from build123d import *

# Parameters (mm, degrees)
SKETCH1_R           = 3.4
BOSS_EXTRUDE1_DEPTH = 400


with BuildPart() as part:
    # Sketch1 → Boss-Extrude1 (new body)
    with BuildSketch(Plane.XY):
        with BuildLine():
            Line((20, 17.75), (20, 5.15))
            Line((20, 5.15), (19, 5.15))
            Line((19, 5.15), (19, 4.15))
            Line((19, 4.15), (15.4, 4.15))
            Line((15.4, 4.15), (15.4, 6.35))
            Line((15.4, 6.35), (16.95, 6.35))
            ThreePointArc((16.95, 6.35), (17.833883476, 6.716116524), (18.2, 7.6))
            Line((18.2, 7.6), (18.2, 9.3))
            ThreePointArc((18.2, 9.3), (17.907106781, 10.007106781), (17.2, 10.3))
            Line((17.2, 10.3), (12.03669957, 10.3))
            ThreePointArc((12.03669957, 10.3), (11.73040037, 10.239040459), (11.470780817, 10.065452001))
            Line((11.470780817, 10.065452001), (6.084081247, 4.674305984))
            ThreePointArc((6.084081247, 4.674305984), (5.910833239, 4.414848262), (5.85, 4.108853983))
            Line((5.85, 4.108853983), (5.85, -4.108853983))
            ThreePointArc((5.85, -4.108853983), (5.910833239, -4.414848262), (6.084081247, -4.674305984))
            Line((6.084081247, -4.674305984), (11.470780817, -10.065452001))
            ThreePointArc((11.470780817, -10.065452001), (11.73040037, -10.239040459), (12.03669957, -10.3))
            Line((12.03669957, -10.3), (17.2, -10.3))
            ThreePointArc((17.2, -10.3), (17.907106781, -10.007106781), (18.2, -9.3))
            Line((18.2, -9.3), (18.2, -7.6))
            ThreePointArc((18.2, -7.6), (17.833883476, -6.716116524), (16.95, -6.35))
            Line((16.95, -6.35), (15.4, -6.35))
            Line((15.4, -6.35), (15.4, -4.15))
            Line((15.4, -4.15), (19, -4.15))
            Line((19, -4.15), (19, -5.15))
            Line((19, -5.15), (20, -5.15))
            Line((20, -5.15), (20, -17.75))
            ThreePointArc((20, -17.75), (19.340990258, -19.340990258), (17.75, -20))
            Line((17.75, -20), (5.15, -20))
            Line((5.15, -20), (5.15, -19))
            Line((5.15, -19), (4.15, -19))
            Line((4.15, -19), (4.15, -15.4))
            Line((4.15, -15.4), (6.35, -15.4))
            Line((6.35, -15.4), (6.35, -16.95))
            ThreePointArc((6.35, -16.95), (6.716116524, -17.833883476), (7.6, -18.2))
            Line((7.6, -18.2), (9.3, -18.2))
            ThreePointArc((9.3, -18.2), (10.007106781, -17.907106781), (10.3, -17.2))
            Line((10.3, -17.2), (10.3, -12.054477022))
            ThreePointArc((10.3, -12.054477022), (10.239166761, -11.748482743), (10.065918753, -11.489025021))
            Line((10.065918753, -11.489025021), (4.665899173, -6.084547999))
            ThreePointArc((4.665899173, -6.084547999), (4.406279619, -5.910959541), (4.09998042, -5.85))
            Line((4.09998042, -5.85), (-4.09998042, -5.85))
            ThreePointArc((-4.09998042, -5.85), (-4.406279619, -5.910959541), (-4.665899173, -6.084547999))
            Line((-4.665899173, -6.084547999), (-10.065918753, -11.489025021))
            ThreePointArc((-10.065918753, -11.489025021), (-10.239166761, -11.748482743), (-10.3, -12.054477022))
            Line((-10.3, -12.054477022), (-10.3, -17.2))
            ThreePointArc((-10.3, -17.2), (-10.007106781, -17.907106781), (-9.3, -18.2))
            Line((-9.3, -18.2), (-7.6, -18.2))
            ThreePointArc((-7.6, -18.2), (-6.716116524, -17.833883476), (-6.35, -16.95))
            Line((-6.35, -16.95), (-6.35, -15.4))
            Line((-6.35, -15.4), (-4.15, -15.4))
            Line((-4.15, -15.4), (-4.15, -19))
            Line((-4.15, -19), (-5.15, -19))
            Line((-5.15, -19), (-5.15, -20))
            Line((-5.15, -20), (-17.75, -20))
            ThreePointArc((-17.75, -20), (-19.340990258, -19.340990258), (-20, -17.75))
            Line((-20, -17.75), (-20, -5.15))
            Line((-20, -5.15), (-19, -5.15))
            Line((-19, -5.15), (-19, -4.15))
            Line((-19, -4.15), (-15.4, -4.15))
            Line((-15.4, -4.15), (-15.4, -6.35))
            Line((-15.4, -6.35), (-16.95, -6.35))
            ThreePointArc((-16.95, -6.35), (-17.833883476, -6.716116524), (-18.2, -7.6))
            Line((-18.2, -7.6), (-18.2, -9.3))
            ThreePointArc((-18.2, -9.3), (-17.907106781, -10.007106781), (-17.2, -10.3))
            Line((-17.2, -10.3), (-12.03669957, -10.3))
            ThreePointArc((-12.03669957, -10.3), (-11.73040037, -10.239040459), (-11.470780817, -10.065452001))
            Line((-11.470780817, -10.065452001), (-6.084081247, -4.674305984))
            ThreePointArc((-6.084081247, -4.674305984), (-5.910833239, -4.414848262), (-5.85, -4.108853983))
            Line((-5.85, -4.108853983), (-5.85, 4.108853983))
            ThreePointArc((-5.85, 4.108853983), (-5.910833239, 4.414848262), (-6.084081247, 4.674305984))
            Line((-6.084081247, 4.674305984), (-11.470780817, 10.065452001))
            ThreePointArc((-11.470780817, 10.065452001), (-11.73040037, 10.239040459), (-12.03669957, 10.3))
            Line((-12.03669957, 10.3), (-17.2, 10.3))
            ThreePointArc((-17.2, 10.3), (-17.907106781, 10.007106781), (-18.2, 9.3))
            Line((-18.2, 9.3), (-18.2, 7.6))
            ThreePointArc((-18.2, 7.6), (-17.833883476, 6.716116524), (-16.95, 6.35))
            Line((-16.95, 6.35), (-15.4, 6.35))
            Line((-15.4, 6.35), (-15.4, 4.15))
            Line((-15.4, 4.15), (-19, 4.15))
            Line((-19, 4.15), (-19, 5.15))
            Line((-19, 5.15), (-20, 5.15))
            Line((-20, 5.15), (-20, 17.75))
            ThreePointArc((-20, 17.75), (-19.340990258, 19.340990258), (-17.75, 20))
            Line((-17.75, 20), (-5.15, 20))
            Line((-5.15, 20), (-5.15, 19))
            Line((-5.15, 19), (-4.15, 19))
            Line((-4.15, 19), (-4.15, 15.4))
            Line((-4.15, 15.4), (-6.35, 15.4))
            Line((-6.35, 15.4), (-6.35, 16.95))
            ThreePointArc((-6.35, 16.95), (-6.716116524, 17.833883476), (-7.6, 18.2))
            Line((-7.6, 18.2), (-9.3, 18.2))
            ThreePointArc((-9.3, 18.2), (-10.007106781, 17.907106781), (-10.3, 17.2))
            Line((-10.3, 17.2), (-10.3, 12.054477022))
            ThreePointArc((-10.3, 12.054477022), (-10.239166761, 11.748482743), (-10.065918753, 11.489025021))
            Line((-10.065918753, 11.489025021), (-4.665899173, 6.084547999))
            ThreePointArc((-4.665899173, 6.084547999), (-4.406279619, 5.910959541), (-4.09998042, 5.85))
            Line((-4.09998042, 5.85), (4.09998042, 5.85))
            ThreePointArc((4.09998042, 5.85), (4.406279619, 5.910959541), (4.665899173, 6.084547999))
            Line((4.665899173, 6.084547999), (10.065918753, 11.489025021))
            ThreePointArc((10.065918753, 11.489025021), (10.239166761, 11.748482743), (10.3, 12.054477022))
            Line((10.3, 12.054477022), (10.3, 17.2))
            ThreePointArc((10.3, 17.2), (10.007106781, 17.907106781), (9.3, 18.2))
            Line((9.3, 18.2), (7.6, 18.2))
            ThreePointArc((7.6, 18.2), (6.716116524, 17.833883476), (6.35, 16.95))
            Line((6.35, 16.95), (6.35, 15.4))
            Line((6.35, 15.4), (4.15, 15.4))
            Line((4.15, 15.4), (4.15, 19))
            Line((4.15, 19), (5.15, 19))
            Line((5.15, 19), (5.15, 20))
            Line((5.15, 20), (17.75, 20))
            ThreePointArc((17.75, 20), (19.340990258, 19.340990258), (20, 17.75))
        make_face()
        Circle(SKETCH1_R, mode=Mode.SUBTRACT)
        with BuildLine():
            Line((18.6, 16.35), (18.6, 12.2))
            ThreePointArc((18.6, 12.2), (18.365685425, 11.634314575), (17.8, 11.4))
            Line((17.8, 11.4), (12.2, 11.4))
            ThreePointArc((12.2, 11.4), (11.634314575, 11.634314575), (11.4, 12.2))
            Line((11.4, 12.2), (11.4, 17.8))
            ThreePointArc((11.4, 17.8), (11.634314575, 18.365685425), (12.2, 18.6))
            Line((12.2, 18.6), (16.35, 18.6))
            ThreePointArc((16.35, 18.6), (17.940990258, 17.940990258), (18.6, 16.35))
        make_face(mode=Mode.SUBTRACT)
        with BuildLine():
            Line((-12.2, 18.6), (-16.35, 18.6))
            ThreePointArc((-16.35, 18.6), (-17.940990258, 17.940990258), (-18.6, 16.35))
            Line((-18.6, 16.35), (-18.6, 12.2))
            ThreePointArc((-18.6, 12.2), (-18.365685425, 11.634314575), (-17.8, 11.4))
            Line((-17.8, 11.4), (-12.2, 11.4))
            ThreePointArc((-12.2, 11.4), (-11.634314575, 11.634314575), (-11.4, 12.2))
            Line((-11.4, 12.2), (-11.4, 17.8))
            ThreePointArc((-11.4, 17.8), (-11.634314575, 18.365685425), (-12.2, 18.6))
        make_face(mode=Mode.SUBTRACT)
        with BuildLine():
            Line((-18.6, -16.35), (-18.6, -12.2))
            ThreePointArc((-18.6, -12.2), (-18.365685425, -11.634314575), (-17.8, -11.4))
            Line((-17.8, -11.4), (-12.2, -11.4))
            ThreePointArc((-12.2, -11.4), (-11.634314575, -11.634314575), (-11.4, -12.2))
            Line((-11.4, -12.2), (-11.4, -17.8))
            ThreePointArc((-11.4, -17.8), (-11.634314575, -18.365685425), (-12.2, -18.6))
            Line((-12.2, -18.6), (-16.35, -18.6))
            ThreePointArc((-16.35, -18.6), (-17.940990258, -17.940990258), (-18.6, -16.35))
        make_face(mode=Mode.SUBTRACT)
        with BuildLine():
            Line((12.2, -18.6), (16.35, -18.6))
            ThreePointArc((16.35, -18.6), (17.940990258, -17.940990258), (18.6, -16.35))
            Line((18.6, -16.35), (18.6, -12.2))
            ThreePointArc((18.6, -12.2), (18.365685425, -11.634314575), (17.8, -11.4))
            Line((17.8, -11.4), (12.2, -11.4))
            ThreePointArc((12.2, -11.4), (11.634314575, -11.634314575), (11.4, -12.2))
            Line((11.4, -12.2), (11.4, -17.8))
            ThreePointArc((11.4, -17.8), (11.634314575, -18.365685425), (12.2, -18.6))
        make_face(mode=Mode.SUBTRACT)
    extrude(amount=BOSS_EXTRUDE1_DEPTH)


solid = part.part
Check sheet for the modelled part. Datum: model origin and axes. Units: mm. A direction names the side the tool comes from. Round coordinates to 2 decimals unless told otherwise and drop trailing zeros. Loops run counter-clockwise (first coordinate to the right, second up) from the corner with the lowest first, then second, coordinate; pieces in that order, holes last.
1. Set-up check for faces 1 (the flat face through (0, -5.85, 197)), 2 (the flat face through (5.85, 0, 197)), 3 (the flat face through (0, 5.85, 197)), 4 (the flat face through (-20, 11, 197)): record each of +Z, -Z, +X, -X, +Y, -Y from which the full face is reachable in a straight line by a thin tool's end or side.
2. Sectioned sample at A-A on x = 0. Record the boundary of the cut face in (y, z).
3. Sectioned sample at C-C on z = 169. Give the number of separate pieces and of enclosed holes in the cut face, and give its area (3 significant figures).
4. Gauge pin test, flat ends, axial feed: pin 1 Ø0.5 at (x, z) = (4.5, 106.5) entering from -Y; pin 2 Ø0.5 at (y, z) = (-19.5, 124) entering from +X; pin 3 Ø2 at (x, z) = (-2, 171.5) entering from +Y. Record the tip position at first contact, or that the pin passes through.
5. Scan lines: probe 1 along Y at (x, z) = (12, 255.5); probe 2 along Y at (x, z) = (-15.5, 67); probe 3 along X at (y, z) = (-5, 372). Record each from-to range of solid material in increasing order.
6. Mould release check, pull along Y, two halves, no side actions. Record for faces 5 (the flat face through (3, 2, 400)), 6 (the flat face through (-11, -20, 197)), 7 (the flat face through (-5.85, 0, 197)): released by +Y, released by -Y, zero draft, split by the parting line, or undercut.
Recorded:
1. face 1: +Z, -Z, -Y
1. face 2: +Z, -Z, +X
1. face 3: +Z, -Z, +Y
1. face 4: +Z, -Z, -X, +Y, -Y
2. outline: (-5.85, 0) - (-3.4, 0) - (-3.4, 400) - (-5.85, 400) - close; (3.4, 0) - (5.85, 0) - (5.85, 400) - (3.4, 400) - close
3. separate pieces: 1
3. enclosed holes: 5
3. area: 464 mm2
4. pin 1: stops at y = -19
4. pin 2: stops at x = 19.43
4. pin 3: stops at y = 5.85
5. probe 1: y = -20 to -18.57, -11.43 to -10.3, 10.3 to 11.43, 18.57 to 20
5. probe 2: y = -20 to -18.6, -11.4 to -10.3, -6.35 to -4.15, 4.15 to 6.35, 10.3 to 11.4, 18.6 to 20
5. probe 3: x = -19 to -15.4, -6.41 to 6.41, 15.4 to 19
6. face 5: zero draft
6. face 6: released by -Y
6. face 7: undercut
